```python
from build123d import *

# Parameters (mm, degrees)
SKETCH_1_W      = 44
SKETCH_1_H      = 6
SKETCH_1_R      = 1.55
EXTRUDE_1_DEPTH = 1.5
SKETCH_2_W      = 44
SKETCH_2_H      = 1.5
EXTRUDE_2_DEPTH = 1.5
SKETCH_4_W      = 44
SKETCH_4_H      = 1.5
EXTRUDE_3_DEPTH = 30
SKETCH_6_W      = 30
SKETCH_6_H      = 1.5
EXTRUDE_4_DEPTH = 50


with BuildPart() as part:
    # 草图1 → 凸台-拉伸1 (new body)
    with BuildSketch(Plane.XY):
        Rectangle(SKETCH_1_W, SKETCH_1_H)
        with Locations((-19.14418972, 0)):
            Circle(SKETCH_1_R, mode=Mode.SUBTRACT)
        with Locations((19.14418972, 0)):
            Circle(SKETCH_1_R, mode=Mode.SUBTRACT)
    extrude(amount=EXTRUDE_1_DEPTH)

    # 草图2 → 凸台-拉伸2 (add)
    with BuildSketch(Plane(origin=(0, 3, 0), x_dir=(1, 0, 0), z_dir=(0, 1, 0))):
        with Locations((0, -0.75)):
            Rectangle(SKETCH_2_W, SKETCH_2_H)
    extrude(amount=EXTRUDE_2_DEPTH)

    # 草图4 → 凸台-拉伸3 (add)
    with BuildSketch(Plane(origin=(0, 0, 0), x_dir=(-1, 0, 0), z_dir=(0, 0, -1))):
        with Locations((0, 3.75)):
            Rectangle(SKETCH_4_W, SKETCH_4_H)
    extrude(amount=EXTRUDE_3_DEPTH)

    # 草图6 → 凸台-拉伸4 (add)
    with BuildSketch(Plane.ZY.offset(22)):
        with Locations((-15, 3.75)):
            Rectangle(SKETCH_6_W, SKETCH_6_H)
    extrude(amount=EXTRUDE_4_DEPTH)


solid = part.part
```
Work out the finished part from the listing and answer in its coordinate system (mm). A direction names the side the tool comes from. Coordinates: 2 decimals unless noted, no trailing zeros. Write each loop counter-clockwise with the first axis right and the second up, starting at its lowest first coordinate (ties: lowest second). Pieces come first, ordered by that corner, then holes.
Q1. Find the intervals of material crossed by line 1 (Y direction, x = -59, z = -9); line 2 (Z direction, x = -3.5, y = 1.25); line 3 (Z direction, x = -28.5, y = 4), in increasing order.
Q2. Each of these flat-tipped pins is pushed along its axis until it touches: pin 1 Ø12 at (x, z) = (3, -6.5) entering from -Y; pin 2 Ø1.5 at (x, y) = (-58.5, 0.5) entering from +Z; pin 3 Ø3.5 at (x, y) = (-19.14, 0) entering from -Z; pin 4 Ø1.2 at (x, y) = (-58, 4) entering from +Z. Where does it stop, or does it pass through?
Q3. A cutting plane is placed at B-B, the plane z = -1. Give the vertices of the cut face in (x, y).
Q4. A cutting plane is placed at A-A, the plane y = 0. Give the vertices of the cut face in (x, z).
Q5. Determine the mould class of faces 4 (the face through (-24, 3, -15)), 5 (the face through (17.596, 0.068, 0.74)), 6 (the face through (-24, 4.5, -14)) for opening direction Y: released by +Y, released by -Y, zero draft, split by the parting line, or undercut.
Q6. A cutting plane is placed at C-C, the plane x = -53.5. Give the vertices of the cut face in (y, z).
Q7. Which of the six approach directions +Z, -Z, +X, -X, +Y, -Y give full straight-line access (tool end or side, diameter ignored) to faces 1 (the face through (-24, 4, -30)), 2 (the face through (-22, 1, 1)), 3 (the face through (0, 0, 0))?
Findings below:
1. line 1: y = 3 to 4.5
1. line 2: z = 0 to 1.5
1. line 3: z = -30 to 0
2. pin 1: stops at y = 3
2. pin 2: passes through
2. pin 3: stops at z = 0
2. pin 4: stops at z = 0
3. outline: (-72, 3) - (22, 3) - (22, 4.5) - (-72, 4.5) - close
4. outline: (-22, 0) - (-20.69, 0) - (-20.69, 1.5) - (-22, 1.5) - close; (-17.59, 0) - (17.59, 0) - (17.59, 1.5) - (-17.59, 1.5) - close; (20.69, 0) - (22, 0) - (22, 1.5) - (20.69, 1.5) - close
5. face 4: released by -Y
5. face 5: undercut
5. face 6: released by +Y
6. outline: (3, -30) - (4.5, -30) - (4.5, 0) - (3, 0) - close
7. face 1: -Z, +X, -X, +Y, -Y
7. face 2: +Z, -X, +Y, -Y
7. face 3: -Z, +X, -X, -Y
